Part print with two shaded views. Sizes in mm from the minimum x, y, z corner. A direction names the side the tool comes from. Round coordinates to 2 decimals unless told otherwise and drop trailing zeros. Loops run counter-clockwise (first coordinate to the right, second up) from the corner with the lowest first, then second, coordinate; pieces in that order, holes last. Notation, with made-up numbers: (27.25, 72) - (71.25, 72) arc R11 cw to (71.25, 88) - close; hole circle Ø9 at (-16, 61). An arc over 180 degrees is marked (long way). Put each result on its own line as item: value. Start each with the question number.
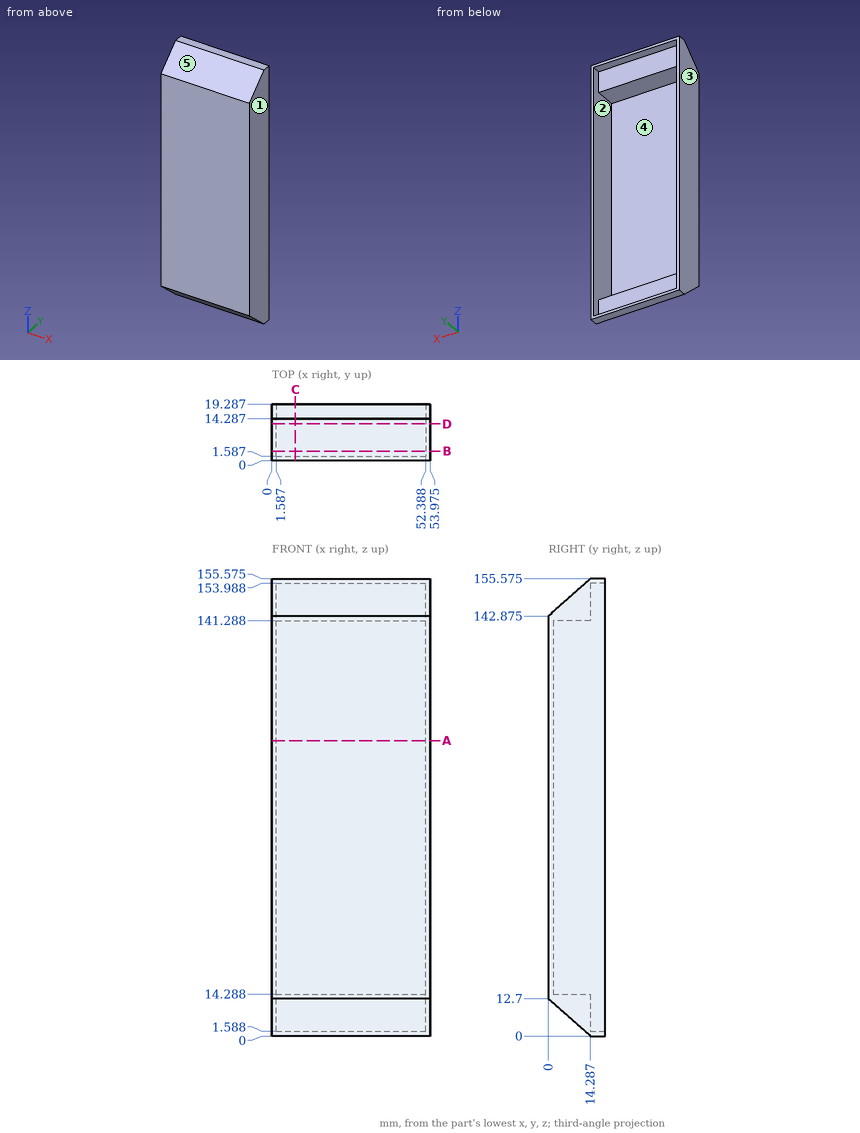
1) Slice it at C-C, the plane x = 8. Write the cut outline in (y, z) (1 decimal).
2) Slice it at D-D, the plane y = 12.5. Write the cut outline in (x, z) (1 decimal).
3) Slice it at B-B, the plane y = 3.25. Write the cut outline in (x, z) (1 decimal).
4) Drill centre lines: line 1 (Z direction, x = 50, y = 16) (1 decimal); line 2 (X direction, y = 18, z = 48) (1 decimal); line 3 (Z direction, x = 19.5, y = 14.25) (1 decimal). Where is each one in solid material? Low to high. Write a range as [from, to].
5) Drop flat-ended pins along their axis: pin 1 Ø1 at (x, z) = (23, 38.5) entering from +Y; pin 2 Ø4 at (x, z) = (32.5, 5) entering from +Y; pin 3 Ø4 at (x, y) = (29, 9) entering from +Z. Give the stop position or say it passes through.
6) Which spindle directions (+Z, -Z, +X, -X, +Y, -Y) get a long thin tool onto all of the face, cutting with end or side? Do the marked faces 4 and 5. Say none if no direction does.
7) Slice it at A-A, the plane z = 100.5. Write the cut outline in (x, y) (1 decimal).
8) Pull direction X, two halves, no side cores. Call the marked faces 1, 2 and 3: pulls with the +X half, pulls with the -X half, needs draft (parallel to the pull), parting line crosses it, or undercut.
Taken from the geometry:
1. outline: (0, 12.7) - (14.3, 0) - (19.3, 0) - (19.3, 1.6) - (14.3, 1.6) - (14.3, 14.3) - (1.6, 14.3) - (1.6, 141.3) - (14.3, 141.3) - (14.3, 154) - (19.3, 154) - (19.3, 155.6) - (14.3, 155.6) - (0, 142.9) - close
2. outline: (0, 1.6) - (54, 1.6) - (54, 154) - (0, 154) - close; hole (1.6, 14.3) - (52.4, 14.3) - (52.4, 141.3) - (1.6, 141.3) - close
3. outline: (0, 9.8) - (54, 9.8) - (54, 145.8) - (0, 145.8) - close; hole (1.6, 14.3) - (52.4, 14.3) - (52.4, 141.3) - (1.6, 141.3) - close
4. line 1: z = [0, 1.6], [154, 155.6]
4. line 2: x = [0, 1.6], [52.4, 54]
4. line 3: z = [0, 14.3], [141.3, 155.5]
5. pin 1: stops at y = 1.59
5. pin 2: stops at y = 14.29
5. pin 3: stops at z = 152.65
6. face 4: +Y
6. face 5: +Z, +X, -X, -Y
7. outline: (0, 0) - (54, 0) - (54, 19.3) - (52.4, 19.3) - (52.4, 1.6) - (1.6, 1.6) - (1.6, 19.3) - (0, 19.3) - close
8. face 1: pulls with the +X half
8. face 2: undercut
8. face 3: pulls with the -X half
